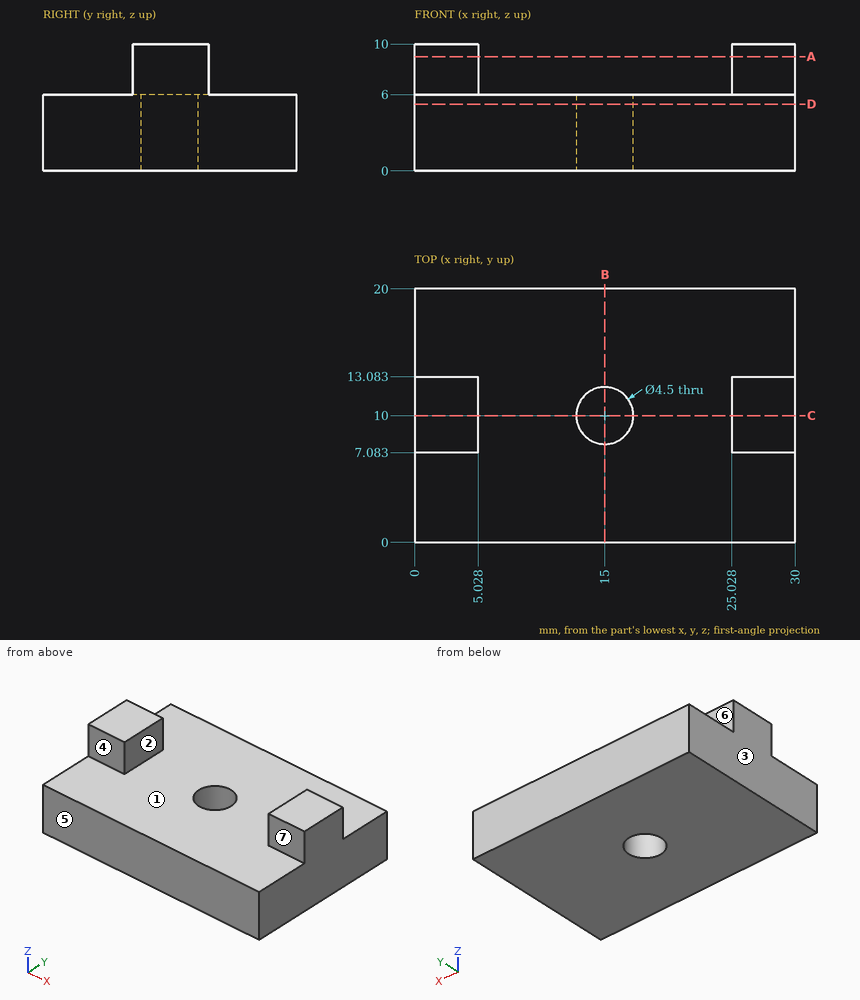
Study the drawing (mm; zero at the part's minimum x, y, z) and answer. A direction names the side the tool comes from. Coordinates: 2 decimals unless noted, no trailing zeros. Write each loop counter-clockwise with the first axis right and the second up, starting at its lowest first coordinate (ties: lowest second). Pieces come first, ordered by that corner, then holes. Notation, with made-up numbers: M 32.25,35.25 L 42.25,35.25 A15 ccw 42.25,63.25 Z; hole C -39,-12.5 d4. An arc over 180 degrees is marked long. Use a Markdown table: item, result. Add a question column.
1. Section B-B (x = 15) is taken. Give the vertices of the cut face in (y, z), plus the area to 3 significant figures.
2. Section A-A (z = 9) is taken. Give the vertices of the cut face in (x, y), plus the area to 3 significant figures.
3. Which of the six approach directions +Z, -Z, +X, -X, +Y, -Y give full straight-line access (tool end or side, diameter ignored) to the marked faces 5, 6 and 7?
4. For a pull along X with two mould halves and no side action, classify the marked faces 1, 2, 3 and 4 as +X half, -X half, draft (parallel to the pull), parting line (faces both ways), or undercut.
5. Section C-C (y = 10) is taken. Give the vertices of the cut face in (x, z).
6. Straight lines are drawn through the part: line 1 along X through (y, z) = (10, 3); line 2 along X through (y, z) = (9, 8); line 3 along Y through (x, z) = (15, 2.95). For each, find the intervals that lie inside material, in ascending order. Write a range as [from, to].
7. Section D-D (z = 5.25) is taken. Give the vertices of the cut face in (x, y), plus the area to 3 significant figures.
8. Given P1, Ø1.2, axis at x = 27.5, z = 8.5, coming from the +Y side; P2, Ø1.5, axis at y = 3, z = 8.5, coming from the -X side; P3, Ø1.2, axis at x = 27, z = 8, coming from the -Y side; P4, Ø6, axis at x = 11.5, y = 8, coming from the +Z side, each flat-ended and moving along its own axis, determine where each tip first touches the part or whether it passes through.
Data:
| question | item | result |
|---|---|---|
| 1 | outline | M 0,0 L 7.75,0 L 7.75,6 L 0,6 Z; M 12.25,0 L 20,0 L 20,6 L 12.25,6 Z |
| 1 | area | 93.0 mm2 |
| 2 | outline | M 0,7.08 L 5.03,7.08 L 5.03,13.08 L 0,13.08 Z; M 25.03,7.08 L 30,7.08 L 30,13.08 L 25.03,13.08 Z |
| 2 | area | 60.0 mm2 |
| 3 | face 5 | +Z, -Z, +X, -X, -Y |
| 3 | face 6 | +Z, +X, -X, +Y |
| 3 | face 7 | +Z, +X, -X, -Y |
| 4 | face 1 | undercut |
| 4 | face 2 | undercut |
| 4 | face 3 | -X half |
| 4 | face 4 | draft |
| 5 | outline | M 0,0 L 12.75,0 L 12.75,6 L 5.03,6 L 5.03,10 L 0,10 Z; M 17.25,0 L 30,0 L 30,10 L 25.03,10 L 25.03,6 L 17.25,6 Z |
| 6 | line 1 | x = [0, 12.75], [17.25, 30] |
| 6 | line 2 | x = [0, 5.03], [25.03, 30] |
| 6 | line 3 | y = [0, 7.75], [12.25, 20] |
| 7 | outline | M 0,0 L 30,0 L 30,20 L 0,20 Z; hole C 15,10 d4.5 |
| 7 | area | 584 mm2 |
| 8 | P1 | stops at y = 13.08 |
| 8 | P2 | passes through |
| 8 | P3 | stops at y = 7.08 |
| 8 | P4 | stops at z = 6 |
